Autodesk Inventor part; units mm, degrees
ref_plane "YZ Plane" through (0, 0, 0) normal (1, 0, 0) x (0, 1, 0)
ref_plane "XZ Plane" through (0, 0, 0) normal (0, 1, 0) x (-1, 0, 0)
ref_plane "XY Plane" through (0, 0, 0) normal (0, 0, 1) x (1, 0, 0)
ref_plane "Arbeitsebene1" through (16.6353, -6.4369, 0) normal (0, 0, 1) x (1, 0, 0)
sketch "Skizze1" plane through (16.6353, -6.4369, 0) normal (0, 0, 1) x (1, 0, 0)
  circle A0 centre (-16.6375, -8.7) radius 1.3
  circle A1 centre (-16.6375, 8.7) radius 1.3
  circle A2 centre (23.3088, -8.7) radius 1.3
  circle A3 centre (23.3715, 8.7) radius 1.3
  point P0 (-16.6353, 6.4369)
extrude "Extrusion1" add sketch "Skizze1" along normal mid plane 4
ref_plane "Arbeitsebene3" through (16.6353, -6.4369, 0) normal (0, 0, 1) x (1, 0, 0)
sketch "Skizze11" plane through (16.6353, -6.4369, 0) normal (0, 0, 1) x (1, 0, 0)
  line L0 (19.6375, -11.7) -> (-19.6375, -11.7)
  line L1 (-19.6375, -11.7) -> (-19.6375, 11.7)
  line L2 (-20.6375, 12.7) -> (27.3715, 12.7)
  line L3 (-19.6375, 11.7) -> (-19.6375, -11.7)
  line L4 (-19.6375, -11.7) -> (26.3715, -11.7)
  line L5 (26.3715, -11.7) -> (26.3715, 11.7)
  line L6 (-19.6375, 11.7) -> (26.3715, 11.7)
  line L7 (-20.6375, -12.7) -> (27.3715, -12.7)
  line L8 (27.3715, -12.7) -> (27.3715, 12.7)
  line L9 (-20.6375, -12.7) -> (27.3715, -12.7)
  line L10 (27.3715, -12.7) -> (27.3715, 12.7)
  line L11 (27.3715, 12.7) -> (-20.6375, 12.7)
  line L12 (-20.6375, 12.7) -> (-20.6375, -12.7)
  point P0 (-16.6353, 6.4369)
  point P1 (19.6375, -11.7)
sketch "Skizze12" plane through (16.6353, -6.4369, 2) normal (0, 0, 1) x (1, 0, 0)
  line L0 (20.6375, 12.7) -> (-20.6375, 12.7)
  line L1 (-20.6375, 12.7) -> (-20.6375, -12.7)
  line L2 (-20.6375, -12.7) -> (20.6375, -12.7)
  line L3 (20.6375, -12.7) -> (20.6375, 12.7)
  circle A0 centre (0, 0) radius 32
  line L4 (20.6375, 12.7) -> (29.3719, 12.7)
  line L5 (29.3719, -12.7) -> (20.6375, -12.7)
  line L6 (29.3719, -12.7) -> (29.3719, 12.7)
  point P0 (-16.6353, 6.4369)
  dimension "d20" = 64
extrude "Extrusion7" add sketch "Skizze12" along normal blind 2 contours L3 L2 L1 L0 | L4 L6 L5 L3 | L0 L1 L2 L5 A0 L4
sketch "Skizze13" plane through (16.6353, -6.4369, 2) normal (0, 0, -1) x (-1, 0, 0)
  arc A0 (-29.3719, -12.7) -> (-29.3719, 12.7) centre (0, 0) ccw
  line L0 (-29.3719, -12.7) -> (-29.3719, 12.7)
  arc A1 (-27.3719, -12.2792) -> (-27.3719, 12.2792) centre (0, 0) ccw
  line L1 (-27.3719, -12.2792) -> (-27.3719, 12.2792)
  point P0 (16.6353, 6.4369)
  dimension "d23" = 2
extrude "Extrusion8" add sketch "Skizze13" along normal blind 24
sketch "Skizze14" plane through (16.6353, -6.4369, -22) normal (0, 0, -1) x (-1, 0, 0)
  line L0 (-27.3719, -12.2792) -> (-27.3719, 12.2792)
  arc A0 (-27.3719, -12.2792) -> (-27.3719, 12.2792) centre (0, 0) ccw
  line L1 (-28.1719, 12.4492) -> (-28.1719, -12.4492)
  arc A1 (-28.1719, -12.4492) -> (-28.1719, 12.4492) centre (0, 0) ccw
  point P0 (16.6353, 6.4369)
  dimension "d26" = 0.8
extrude "Extrusion9" add sketch "Skizze14" along normal blind 4
sketch "Skizze18" plane through (46.0073, -19.1369, 4) normal (1, 0, 0) x (0, 0, -1)
  line L0 (18.8305, 15.87) -> (18.8305, 9.53) construction
  line L1 (18.8305, 15.87) -> (18.8305, 12.7)
  line L2 (20.4105, 15.87) -> (20.4105, 9.53) construction
  line L3 (18.8305, 9.53) -> (18.8305, 15.87)
  line L4 (18.8305, 15.87) -> (18.8305, 9.53) construction
  line L5 (20.4105, 15.87) -> (20.4105, 9.53) construction
  line L6 (21.9905, 15.87) -> (21.9905, 9.53)
  line L7 (18.8305, 9.53) -> (18.8305, 15.87)
  arc A0 (21.9905, 15.87) -> (18.8305, 15.87) centre (20.4105, 15.87) ccw
  arc A1 (18.8305, 9.53) -> (21.9905, 9.53) centre (20.4105, 9.53) ccw
  line L8 (23.4905, 9.53) -> (23.4905, 15.87)
  arc A2 (23.4905, 15.87) -> (17.3305, 15.87) centre (20.4105, 15.87) ccw
  line L9 (17.3305, 15.87) -> (17.3305, 9.53)
  arc A3 (17.3305, 9.53) -> (23.4905, 9.53) centre (20.4105, 9.53) ccw
  line L10 (26, 25.4) -> (0, 25.4)
  line L11 (0, 0) -> (26, 0)
  point P0 (4, 19.1369)
  point P1 (20.4105, 12.7)
  point P2 (18.8305, 12.7)
  point P3 (20.4105, 12.7)
  dimension "d75" = 1.5
extrude "Extrusion10" cut sketch "Skizze18" against normal blind 4 contours A0 L6 A1 L3 L1 | A3 L9 A2 L8
sketch "Skizze19" plane through (46.0073, -19.1369, 4) normal (1, 0, 0) x (0, 0, -1)
  arc A0 (14.7505, 9.53) -> (22.9105, 9.53) centre (18.8305, 9.53) ccw
  line L0 (14.7505, 9.53) -> (14.7505, 15.87)
  arc A1 (22.9105, 15.87) -> (14.7505, 15.87) centre (18.8305, 15.87) ccw
  line L1 (0.5305, 7.35) -> (14.0305, 18.05) construction
  line L2 (0.5305, 18.05) -> (14.0305, 7.35) construction
  line L3 (14.3305, 7.05) -> (14.3305, 18.35)
  line L4 (14.3305, 18.35) -> (0.2305, 18.35)
  line L5 (0.2305, 18.35) -> (0.2305, 7.05)
  line L6 (0.2305, 7.05) -> (14.3305, 7.05)
  point P0 (4, 19.1369)
  dimension "d43" = 10.7
  dimension "d44" = 13.5
extrude "Extrusion11" cut sketch "Skizze19" against normal blind 1.2
sketch "Skizze20" plane through (44.8073, -19.1369, 4) normal (1, 0, 0) x (0, 0, -1)
  line L0 (14.3305, 18.35) -> (14.3305, 7.05)
  line L1 (0.2305, 18.35) -> (14.3305, 18.35)
  line L2 (14.3305, 7.05) -> (0.2305, 7.05)
  line L3 (14.3305, 18.35) -> (10.3305, 18.35)
  line L4 (10.3305, 18.35) -> (10.3305, 7.05)
  line L5 (10.3305, 7.05) -> (14.3305, 7.05)
  line L6 (14.3305, 7.05) -> (14.3305, 18.35)
  point P0 (4, 19.1369)
  dimension "d49" = 4
extrude "Extrusion12" cut sketch "Skizze20" against normal blind 1.2
extrude "Extrusion14" add sketch "Skizze11" along normal blind 2
properties part number "Boden"
For this review, take the finished solid that the model builds, in its own axes (mm). A direction names the side the tool comes from. Coordinates: 2 decimals unless noted, no trailing zeros. Write each loop counter-clockwise with the first axis right and the second up, starting at its lowest first coordinate (ties: lowest second). Pieces come first, ordered by that corner, then holes. Notation, with made-up numbers: (84, 22.5) - (134, 22.5) arc R22 cw to (134, 54.5) - close; hole circle Ø5 at (-37.75, 36). An arc over 180 degrees is marked (long way). Put each result on its own line as item: value.
1. Add section A-A, the plane z = -3.25. Give the boundary of the cut face in (x, y).
Values found:
outline: (44.81, -12.09) - (44.81, -0.79) - (46.01, -0.79) - (46.01, 6.26) arc R32 ccw (long way) to (46.01, -19.14) - (46.01, -12.09) - close; hole (44.01, -18.72) - (44.01, 5.84) arc R30 ccw (long way) to start
2. For pin 1 (0.6 mm diameter, centred on x = 45.5, y = -8, fed in from -Z); pin 2 (1.3 mm diameter, centred on x = 0.5, y = -15.5, fed in from -Z); pin 3 (2 mm diameter, centred on x = 45.5, y = -6, fed in from -Z); pin 4 (1.6 mm diameter, centred on x = 12, z = 0.5, fed in from +Y), all flat-tipped, find the tip position at first contact; note any pin that passes through.
Values found:
pin 1: z = -22
pin 2: z = -2
pin 3: z = -26
pin 4: y = 25.33
3. Add section B-B, the plane x = 11.5. Give the boundary of the cut face in (y, z).
Values found:
outline: (-38.02, -22) - (-36.81, -22) - (-36.81, -26) - (-35.99, -26) - (-35.99, 2) - (-19.14, 2) - (-19.14, 0) - (-18.14, 0) - (-18.14, 2) - (5.26, 2) - (5.26, 0) - (6.26, 0) - (6.26, 2) - (23.12, 2) - (23.12, -26) - (23.93, -26) - (23.93, -22) - (25.15, -22) - (25.15, 4) - (-38.02, 4) - close
4. Add section C-C, the plane y = 8. Give the boundary of the cut face in (x, z), then the cut area to 3 significant figures.
Values found:
outline: (-11.92, -22) - (-10.57, -22) - (-10.57, -26) - (-9.66, -26) - (-9.66, 2) - (42.93, 2) - (42.93, -26) - (43.84, -26) - (43.84, -22) - (45.19, -22) - (45.19, 4) - (-11.92, 4) - close
area: 230 mm²
5. Wall thickness on probe 1 along X at (y, z) = (-6.5, -10.5); probe 2 along Y at (x, z) = (17, -15); probe 3 along Z at (x, y) = (10, -8.5): over which ranges is each line inside the solid? List them lowest first.
Values found:
probe 1: -15.36 to -13.36, 44.01 to 46.01
probe 2: -38.43 to -36.43, 23.56 to 25.56
probe 3: 2 to 4
6. Machinability: for faces 4 (the flat face through (40, -15, -2)), 5 (the flat face through (-10.8, -20, -26)), 6 (the flat face through (45, -0.787, -5)), which of the approach directions +Z, -Z, +X, -X, +Y, -Y give a long, thin tool a straight path to every point of the face, cutting with its end or side? Answer none if there is none.
Values found:
face 4: -Z
face 5: -Z, +X, -X, +Y, -Y
face 6: +X
7. Add section D-D, the plane z = -23. Give the boundary of the cut face in (x, y).
Values found:
outline: (44.81, -18.89) - (44.81, 6.01) arc R30.8 ccw (long way) to start; hole (44.01, -18.72) - (44.01, 5.84) arc R30 ccw (long way) to start
8. Mouldability with a two-part tool opening along X and no side actions: class faces 1 (the flat face through (44.807, -6, -24)), 2 (the cylindrical face through (45.021, -0.188, -16.478)), 3 (the flat face through (20, 6.263, 1)) as released by +X, released by -X, zero draft, split by the parting line, or undercut.
Values found:
face 1: released by +X
face 2: zero draft
face 3: undercut
